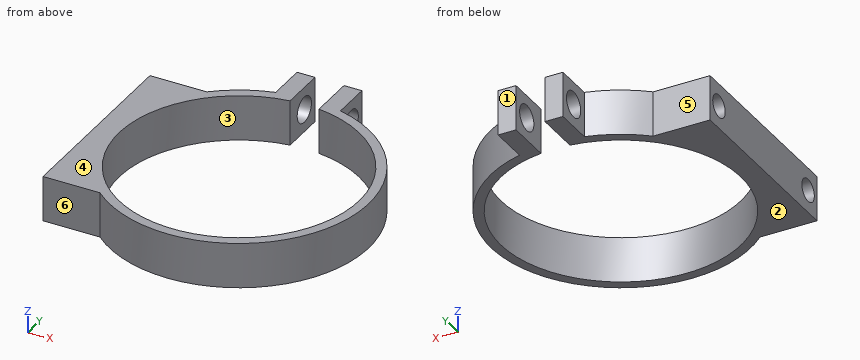
from build123d import *

# Parameters (mm, degrees)
BOSS_EXTRUDE1_DEPTH = 7
SKETCH2_R           = 1.75
CUT_EXTRUDE2_DEPTH  = 5
SKETCH3_R           = 2
CUT_EXTRUDE3_DEPTH  = 15


with BuildPart() as part:
    # Sketch1 → Boss-Extrude1 (new body)
    with BuildSketch(Plane.XY):
        with BuildLine():
            Line((-22, -15), (-22, 15))
            Line((-22, 15), (-13.228756555, 15))
            ThreePointArc((-13.228756555, 15), (-9.372033712, 17.668191308), (-5, 19.364916731))
            Line((-5, 19.364916731), (-5, 25.364916731))
            Line((-5, 25.364916731), (-2.231554046, 25.364916731))
            Line((-2.231554046, 25.364916731), (-2.231554046, 18.364916731))
            ThreePointArc((-2.231554046, 18.364916731), (0, -18.5), (2.231554046, 18.364916731))
            Line((2.231554046, 18.364916731), (2.231554046, 25.364916731))
            Line((2.231554046, 25.364916731), (5, 25.364916731))
            Line((5, 25.364916731), (5, 19.364916731))
            ThreePointArc((5, 19.364916731), (17.668191308, -9.372033712), (-13.228756555, -15))
            Line((-13.228756555, -15), (-22, -15))
        make_face()
    extrude(amount=BOSS_EXTRUDE1_DEPTH)

    # Sketch2 → Cut-Extrude2 (cut)
    with BuildSketch(Plane.ZY.offset(22)):
        with Locations((3.5, 12.5)):
            Circle(SKETCH2_R)
        with Locations((3.5, -12.5)):
            Circle(SKETCH2_R)
    extrude(amount=-CUT_EXTRUDE2_DEPTH, mode=Mode.SUBTRACT)

    # Sketch3 → Cut-Extrude3 (cut)
    with BuildSketch(Plane.ZY.offset(5)):
        with Locations(Location((3.5, 22.364916731, 0), (0, 0, 270))):
            Circle(SKETCH3_R)
    extrude(amount=-CUT_EXTRUDE3_DEPTH, mode=Mode.SUBTRACT)


solid = part.part
Design review of the part built by this model. Coordinates are the model's own, in mm. Face numbers are marked on the shaded views. A direction names the side the tool comes from. Round coordinates to 2 decimals unless told otherwise and drop trailing zeros. Write each loop counter-clockwise with the first axis right and the second up, starting at its lowest first coordinate (ties: lowest second). Pieces come first, ordered by that corner, then holes. Notation, with made-up numbers: (-14, 6) - (26, 6) arc R10 cw to (26, 22) - close; hole circle Ø3 at (27.5, 32). An arc over 180 degrees is marked (long way). Return JSON: item names as keys, results as strings. Group by question number.
Item 1: For probe 1 along Y at (x, z) = (-19.65, 3.5); probe 2 along X at (y, z) = (0, 3.75); probe 3 along Y at (x, z) = (0, 5.5), list the stretches that pass through material, from the lowest coordinate up. Write a range as [from, to].
Item 2: Insertion check: P1, Ø3, axis at y = 23.5, z = 3, coming from the -X side; P2, Ø1, axis at y = 12.5, z = 3, coming from the -X side; P3, Ø1.5, axis at x = 13, z = 4.5, coming from the +Y side. Each pin has a flat end and moves straight along its axis. Give the tip position at first contact, or say it passes through.
Item 3: We need section A-A on y = 0. Write out the cut boundary in (x, z).
Item 4: We need section D-D on x = -4. Write out the cut boundary in (y, z).
Item 5: We need section B-B on x = -9. Write out the cut boundary in (y, z).
Item 6: Machinability: for the marked faces 4, 5 and 6, which of the approach directions +Z, -Z, +X, -X, +Y, -Y give a long, thin tool a straight path to every point of the face, cutting with its end or side? Answer none if there is none.
Item 7: We need section C-C on z = 3. Write out the cut boundary in (x, y), and give its area (3 significant figures).
Item 8: The part is to be moulded in two halves that separate along Y. For the marked faces 1, 2 and 3, say which applies: pulls with the +Y half, pulls with the -Y half, needs draft (parallel to the pull), parting line crosses it, or undercut.
Model answer:
{
 "1": {"probe 1": "y = [-15, -14.25], [-10.75, 10.75], [14.25, 15]", "probe 2": "x = [-22, -18.5], [18.5, 20]", "probe 3": "y = [-20, -18.5]"},
 "2": {"P1": "stops at x = -5", "P2": "stops at x = -17", "P3": "stops at y = 15.81"},
 "3": {"outline": "(-22, 0) - (-18.5, 0) - (-18.5, 7) - (-22, 7) - close; (18.5, 0) - (20, 0) - (20, 7) - (18.5, 7) - close"},
 "4": {"outline": "(-19.6, 0) - (-18.06, 0) - (-18.06, 7) - (-19.6, 7) - close; (18.06, 0) - (25.36, 0) - (25.36, 7) - (18.06, 7) - close; hole circle Ø4 at (22.36, 3.5)"},
 "5": {"outline": "(-17.86, 0) - (-16.16, 0) - (-16.16, 7) - (-17.86, 7) - close; (16.16, 0) - (17.86, 0) - (17.86, 7) - (16.16, 7) - close"},
 "6": {"face 4": "+Z, +X, -X, +Y, -Y", "face 5": "+Z, -Z, -X, +Y", "face 6": "+Z, -Z, -X, -Y"},
 "7": {"outline": "(-22, -15) - (-13.23, -15) arc R20 ccw (long way) to (5, 19.36) - (5, 20.43) - (2.23, 20.43) - (2.23, 18.36) arc R18.5 cw (long way) to (-2.23, 18.36) - (-2.23, 20.43) - (-5, 20.43) - (-5, 19.36) arc R20 ccw to (-13.23, 15) - (-22, 15) - (-22, 14.18) - (-17, 14.18) - (-17, 10.82) - (-22, 10.82) - (-22, -10.82) - (-17, -10.82) - (-17, -14.18) - (-22, -14.18) - close; (-5, 24.3) - (-2.23, 24.3) - (-2.23, 25.36) - (-5, 25.36) - close; (2.23, 24.3) - (5, 24.3) - (5, 25.36) - (2.23, 25.36) - close", "area": "274 mm²"},
 "8": {"face 1": "pulls with the +Y half", "face 2": "needs draft", "face 3": "undercut"}
}
